from build123d import *

# Parameters (mm, degrees)
ESQUISSE1_R                  = 1.7
BOSS_EXTRU_1_DEPTH           = 5
ESQUISSE2_R                  = 3.5
ESQUISSE2_R_2                = 1.7
BOSS_EXTRU_2_DEPTH           = 1
BOSS_EXTRU_3_START           = 9
ESQUISSE5_R                  = 7
BOSS_EXTRU_3_DEPTH           = 9
ESQUISSE6_R                  = 11.5
BOSS_EXTRU_4_DEPTH           = 2
ESQUISSE7_R                  = 4.739811
ENL_V_MAT_EXTRU_1_DEPTH      = 10
ESQUISSE8_R                  = 11.5
ESQUISSE8_R_2                = 6.75
BOSS_EXTRU_5_DEPTH           = 10
ESQUISSE10_R                 = 6.9395
ESQUISSE10_R_2               = 6.2
BOSS_EXTRU_6_DEPTH           = 10
ENL_V_MAT_EXTRU_2_DEPTH      = 28.847054
ENL_V_MAT_EXTRU_2_DEPTH_BACK = 28.847054
ESQUISSE9_R                  = 1.95
BOSS_EXTRU_7_DEPTH           = 4
ESQUISSE12_R                 = 9
ENL_V_MAT_EXTRU_3_DEPTH      = 2


with BuildPart() as part:
    # Esquisse1 → Boss.-Extru.1 (new body)
    with BuildSketch(Plane(origin=(0, 0, 0), x_dir=(1, 0, 0), z_dir=(0, 1, 0))):
        with BuildLine():
            Line((-10.72, 3.5), (-6.062178, 3.5))
            ThreePointArc((-6.062178, 3.5), (0, 7), (6.062178, 3.5))
            Line((6.062178, 3.5), (10.72, 3.5))
            ThreePointArc((10.72, 3.5), (14.22, 0), (10.72, -3.5))
            Line((10.72, -3.5), (6.062178, -3.5))
            ThreePointArc((6.062178, -3.5), (0, -7), (-6.062178, -3.5))
            Line((-6.062178, -3.5), (-10.72, -3.5))
            ThreePointArc((-10.72, -3.5), (-14.22, 0), (-10.72, 3.5))
        make_face()
        with Locations(Location((10.72, 0, 0), (0, 0, 270))):
            Circle(ESQUISSE1_R, mode=Mode.SUBTRACT)
        with Locations(Location((-10.72, 0, 0), (0, 0, 270))):
            Circle(ESQUISSE1_R, mode=Mode.SUBTRACT)
    extrude(amount=BOSS_EXTRU_1_DEPTH)

    # Esquisse2 → Boss.-Extru.2 (add)
    # profile 1 of 2: a face of its own
    with BuildSketch(Plane(origin=(0, 5, 0), x_dir=(1, 0, 0), z_dir=(0, 1, 0))):
        with Locations(Location((-10.72, 0, 0), (0, 0, 270))):
            Circle(ESQUISSE2_R)
        with Locations(Location((-10.72, 0, 0), (0, 0, 270))):
            Circle(ESQUISSE2_R_2, mode=Mode.SUBTRACT)
    # profile 2 of 2: a face of its own
    with BuildSketch(Plane(origin=(0, 5, 0), x_dir=(1, 0, 0), z_dir=(0, 1, 0))):
        with Locations(Location((10.72, 0, 0), (0, 0, 270))):
            Circle(ESQUISSE2_R)
        with Locations(Location((10.72, 0, 0), (0, 0, 270))):
            Circle(ESQUISSE2_R_2, mode=Mode.SUBTRACT)
    extrude(amount=BOSS_EXTRU_2_DEPTH)

    # Esquisse5 → Boss.-Extru.3 (add)
    with BuildSketch(Plane.XZ.offset(BOSS_EXTRU_3_START)):
        with Locations(Location((0, 0, 0), (0, 0, 270))):
            Circle(ESQUISSE5_R)
    extrude(amount=-BOSS_EXTRU_3_DEPTH)

    # Esquisse6 → Boss.-Extru.4 (add)
    with BuildSketch(Plane.XZ.offset(9)):
        with Locations(Location((0, 0, 0), (0, 0, 270))):
            Circle(ESQUISSE6_R)
    extrude(amount=BOSS_EXTRU_4_DEPTH)

    # Esquisse7 → Enlèv. mat.-Extru.1 (cut)
    with BuildSketch(Plane(origin=(0, 5, 0), x_dir=(1, 0, 0), z_dir=(0, 1, 0))):
        with Locations(Location((0, 0, 0), (0, 0, 270))):
            Circle(ESQUISSE7_R)
    extrude(amount=-ENL_V_MAT_EXTRU_1_DEPTH, mode=Mode.SUBTRACT)

    # Esquisse8 → Boss.-Extru.5 (add)
    with BuildSketch(Plane.XZ.offset(11)):
        with Locations(Location((0, 0, 0), (0, 0, 270))):
            Circle(ESQUISSE8_R)
        with Locations(Location((0, 0, 0), (0, 0, 270))):
            Circle(ESQUISSE8_R_2, mode=Mode.SUBTRACT)
    extrude(amount=BOSS_EXTRU_5_DEPTH)

    # Esquisse10 → Boss.-Extru.6 (add)
    with BuildSketch(Plane.XZ.offset(11)):
        Circle(ESQUISSE10_R)
        with Locations(Location((0, 0, 0), (0, 0, 90))):
            Circle(ESQUISSE10_R_2, mode=Mode.SUBTRACT)
    extrude(amount=BOSS_EXTRU_6_DEPTH)

    # Esquisse9 → Enlèv. mat.-Extru.2 (cut, two sides: drawn at the far end of the back side and taken through both)
    with BuildSketch(Plane.XY.offset(-ENL_V_MAT_EXTRU_2_DEPTH_BACK)):
        with Locations(Location((0, -17, 0), (0, 0, 270))):
            Circle(ESQUISSE9_R)
    extrude(amount=ENL_V_MAT_EXTRU_2_DEPTH + ENL_V_MAT_EXTRU_2_DEPTH_BACK, mode=Mode.SUBTRACT)

    # Esquisse11 → Boss.-Extru.7 (add)
    with BuildSketch(Plane.XZ.offset(11)):
        with BuildLine():
            Line((0, 6.2), (6.2, 0))
            ThreePointArc((6.2, 0), (4.384062, 4.384062), (0, 6.2))
        make_face()
    extrude(amount=BOSS_EXTRU_7_DEPTH)

    # Esquisse12 → Enlèv. mat.-Extru.3 (cut)
    with BuildSketch(Plane.XZ.offset(21)):
        with Locations(Location((0, 0, 0), (0, 0, 270))):
            Circle(ESQUISSE12_R)
    extrude(amount=-ENL_V_MAT_EXTRU_3_DEPTH, mode=Mode.SUBTRACT)


solid = part.part
Work out the finished part from the listing and answer in its coordinate system (mm). A direction names the side the tool comes from. Give positions to 0.01 mm unless a question says otherwise; leave off trailing zeros. Loops run counter-clockwise (first coordinate to the right, second up) from the corner with the lowest first, then second, coordinate; pieces in that order, holes last. Notation, with made-up numbers: (80, -30.5) -> (107, -30.5) arc R31 cw to (107, 1.5) -> close; hole circle Ø1 at (30, 36.5). An arc over 180 degrees is marked (long way). Use a Markdown table: item, result. Add a question column.
1. Find the intervals of material crossed by probe 1 along X at (y, z) = (1.25, 0); probe 2 along X at (y, z) = (-20.4, 0); probe 3 along Y at (x, z) = (0, -9.25), in increasing order.
2. Section B-B on y = 3.5 is taken. Determine the outline of the cut face in (x, z).
3. For faces 4 (the cylindrical face through (-9.034, 2.958, -0.221)), 5 (the flat face through (0, -9, -8)), 6 (the flat face through (8, 2, -3.5)), determine the directions among +Z, -Z, +X, -X, +Y, -Y from which every point of the face is accessible in a straight line to the end or side of a thin tool.
4. Section D-D on y = -9.5 is taken. Determine the outline of the cut face in (x, z).
5. Determine the mould class of faces 1 (the cylindrical face through (-13.825, 2.958, 1.615)), 2 (the flat face through (-10, 6, 2)), 3 (the cylindrical face through (0.086, -15.052, -8.732)) for opening direction Y: released by +Y, released by -Y, zero draft, split by the parting line, or undercut.
6. Section C-C on y = -17 is taken. Determine the outline of the cut face in (x, z), and give its area (3 significant figures).
7. Section A-A on x = -9.5 is taken. Determine the outline of the cut face in (y, z).
8. Flat-ended cylindrical pins translate along their axes: pin 1 Ø6 at (x, z) = (-1.5, -2) entering from -Y; pin 2 Ø5 at (x, y) = (5, -9) entering from -Z (3 decimals); pin 3 Ø1.5 at (x, y) = (3.5, -5) entering from -Z. Find the tip coordinate at first contact, or state that the pin passes through.
Results below:
| question | item | result |
|---|---|---|
| 1 | probe 1 | x = -14.22 to -12.42, -9.02 to -4.74, 4.74 to 9.02, 12.42 to 14.22 |
| 1 | probe 2 | x = -11.5 to -9, 9 to 11.5 |
| 1 | probe 3 | y = -21 to -18.95, -15.05 to -9 |
| 2 | outline | (-10.72, -3.5) -> (-6.06, -3.5) arc R7 ccw to (6.06, -3.5) -> (10.72, -3.5) arc R3.5 ccw to (10.72, 3.5) -> (6.06, 3.5) arc R7 ccw to (-6.06, 3.5) -> (-10.72, 3.5) arc R3.5 ccw to start; hole circle Ø3.4 at (-10.72, 0); hole circle Ø9.48 at (0, 0); hole circle Ø3.4 at (10.72, 0) |
| 3 | face 4 | +Y |
| 3 | face 5 | none |
| 3 | face 6 | -Z, +X, +Y |
| 4 | outline | circle Ø23 at (0, 0) |
| 5 | face 1 | zero draft |
| 5 | face 2 | released by +Y |
| 5 | face 3 | undercut |
| 6 | outline | (-1.95, -11.33) -> (-1.95, -5.89) arc R6.2 cw to (-1.95, 5.89) -> (-1.95, 11.33) arc R11.5 ccw to start; (1.95, -11.33) arc R11.5 ccw to (1.95, 11.33) -> (1.95, 5.89) arc R6.2 cw to (1.95, -5.89) -> close |
| 6 | area | 253 mm^2 |
| 7 | outline | (-21, -6.48) -> (-9, -6.48) -> (-9, 6.48) -> (-21, 6.48) -> close; (0, -3.5) -> (5, -3.5) -> (5, -3.28) -> (6, -3.28) -> (6, -1.18) -> (0, -1.18) -> close; (0, 1.18) -> (6, 1.18) -> (6, 3.28) -> (5, 3.28) -> (5, 3.5) -> (0, 3.5) -> close |
| 8 | pin 1 | stops at y = -11 |
| 8 | pin 2 | stops at z = -11.225 |
| 8 | pin 3 | stops at z = -6.44 |
